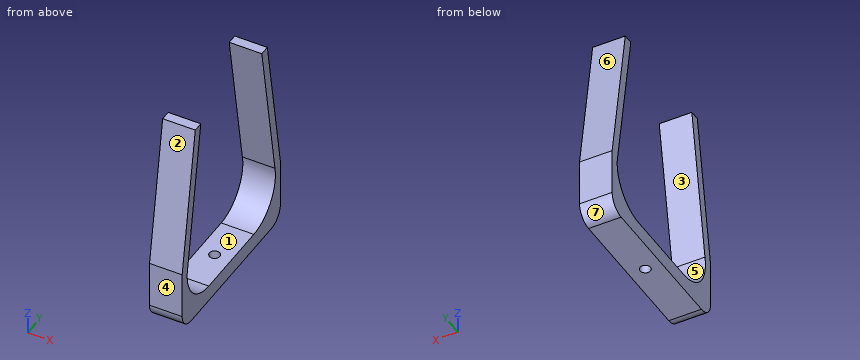
```python
from build123d import *

# Parameters (mm, degrees)
PAD_DEPTH    = 10
FILLET_R     = 5
SKETCH001_R  = 1.6
POCKET_DEPTH = 5.001


with BuildPart() as part:
    # Sketch → Pad (new body)
    with BuildSketch(Plane.YZ):
        with BuildLine():
            Line((-12.5, -14.5), (12.5, -14.5))
            ThreePointArc((12.5, -14.5), (21.827379, -10.049834), (24.236695, 0))
            Line((24.236695, 0), (16.946495, 45))
            Line((16.946495, 45), (20, 45))
            Line((27.290199, 0), (20, 45))
            Line((27.290199, -19.5), (27.290199, 0))
            Line((-27.290199, -19.5), (27.290199, -19.5))
            Line((-27.290199, 0), (-27.290199, -19.5))
            Line((-27.290199, 0), (-20, 45))
            Line((-20, 45), (-16.946495, 45))
            Line((-24.236695, 0), (-16.946495, 45))
            ThreePointArc((-24.236695, 0), (-21.827379, -10.049834), (-12.5, -14.5))
        make_face()
    extrude(amount=PAD_DEPTH)

    # Fillet
    fillet_edges = [part.edges().sort_by_distance(p)[0] for p in [
        (5, -27.290199, -19.5),
        (5, 27.290199, -19.5),
    ]]
    fillet(fillet_edges, radius=FILLET_R)

    # Sketch001 (on Face13 of Fillet) → Pocket (cut, through all)
    with BuildSketch(Plane(origin=(0, 0, -14.5), x_dir=(0, -1, 0), z_dir=(0, 0, 1))):
        with Locations((0.11428, 4.954288)):
            Circle(SKETCH001_R)
    extrude(amount=-POCKET_DEPTH, mode=Mode.SUBTRACT)


solid = part.part
```
Work out the finished part from the listing and answer in its coordinate system (mm). Face numbers are marked on the shaded views. A direction names the side the tool comes from. Give positions to 0.01 mm unless a question says otherwise; leave off trailing zeros. Write each loop counter-clockwise with the first axis right and the second up, starting at its lowest first coordinate (ties: lowest second). Pieces come first, ordered by that corner, then holes.
(1) The part is cut by section B-B on x = 1. Write down the section's boundary in (y, z), plus the area to 3 significant figures.
Final values:
outline: (-27.29, -14.5) arc R5 ccw to (-22.29, -19.5) - (22.29, -19.5) arc R5 ccw to (27.29, -14.5) - (27.29, 0) - (20, 45) - (16.95, 45) - (24.24, 0) arc R12 cw to (12.5, -14.5) - (-12.5, -14.5) arc R12 cw to (-24.24, 0) - (-16.95, 45) - (-20, 45) - (-27.29, 0) - close
area: 680 mm2
(2) The part is cut by section C-C on z = 25. Write down the section's boundary in (x, y).
Final values:
outline: (0, -23.24) - (10, -23.24) - (10, -20.19) - (0, -20.19) - close; (0, 20.19) - (10, 20.19) - (10, 23.24) - (0, 23.24) - close
(3) The mould has two halves that part along Z. Classify the marked faces 4, 5, 6 and 7: pulls with the +Z half, pulls with the -Z half, needs draft (parallel to the pull), parting line crosses it, or undercut.
Final values:
face 4: needs draft
face 5: undercut
face 6: pulls with the +Z half
face 7: pulls with the -Z half
(4) The part is cut by section D-D on x = 4.25. Write down the section's boundary in (y, z).
Final values:
outline: (-27.29, -14.5) arc R5 ccw to (-22.29, -19.5) - (-1.55, -19.5) - (-1.55, -14.5) - (-12.5, -14.5) arc R12 cw to (-24.24, 0) - (-16.95, 45) - (-20, 45) - (-27.29, 0) - close; (1.32, -19.5) - (22.29, -19.5) arc R5 ccw to (27.29, -14.5) - (27.29, 0) - (20, 45) - (16.95, 45) - (24.24, 0) arc R12 cw to (12.5, -14.5) - (1.32, -14.5) - close
(5) Flat-ended cylindrical pins translate along their axes: pin 1 Ø2.5 at (x, y) = (4.95, -0.11) entering from +Z; pin 2 Ø3 at (x, z) = (6, 2.5) entering from +Y; pin 3 Ø4 at (x, z) = (2.5, 23.5) entering from -Y; pin 4 Ø3 at (x, z) = (8.5, 38.5) entering from -Y. Find the tip coordinate at first contact, or state that the pin passes through.
Final values:
pin 1: passes through
pin 2: stops at y = 27.13
pin 3: stops at y = -23.81
pin 4: stops at y = -21.3
(6) Which of the six approach directions +Z, -Z, +X, -X, +Y, -Y give full straight-line access (tool end or side, diameter ignored) to the marked faces 1, 2 and 3?
Final values:
face 1: +Z, +X, -X
face 2: +Z, +X, -X, -Y
face 3: +X, -X
(7) The part is cut by section A-A on y = -21.5. Write down the section's boundary in (x, z).
Final values:
outline: (0, -19.5) - (10, -19.5) - (10, -10.44) - (0, -10.44) - close; (0, 16.89) - (10, 16.89) - (10, 35.74) - (0, 35.74) - close
(8) Straight lines are drawn through the part: line 1 (Y direction, x = 0.5, z = 12.5); line 2 (Z direction, x = 1, y = -2.5); line 3 (Y direction, x = 6, z = 1.5). For each, find the intervals that lie inside material, in ascending order.
Final values:
line 1: y = -25.27 to -22.21, 22.21 to 25.27
line 2: z = -19.5 to -14.5
line 3: y = -27.05 to -23.99, 23.99 to 27.05
